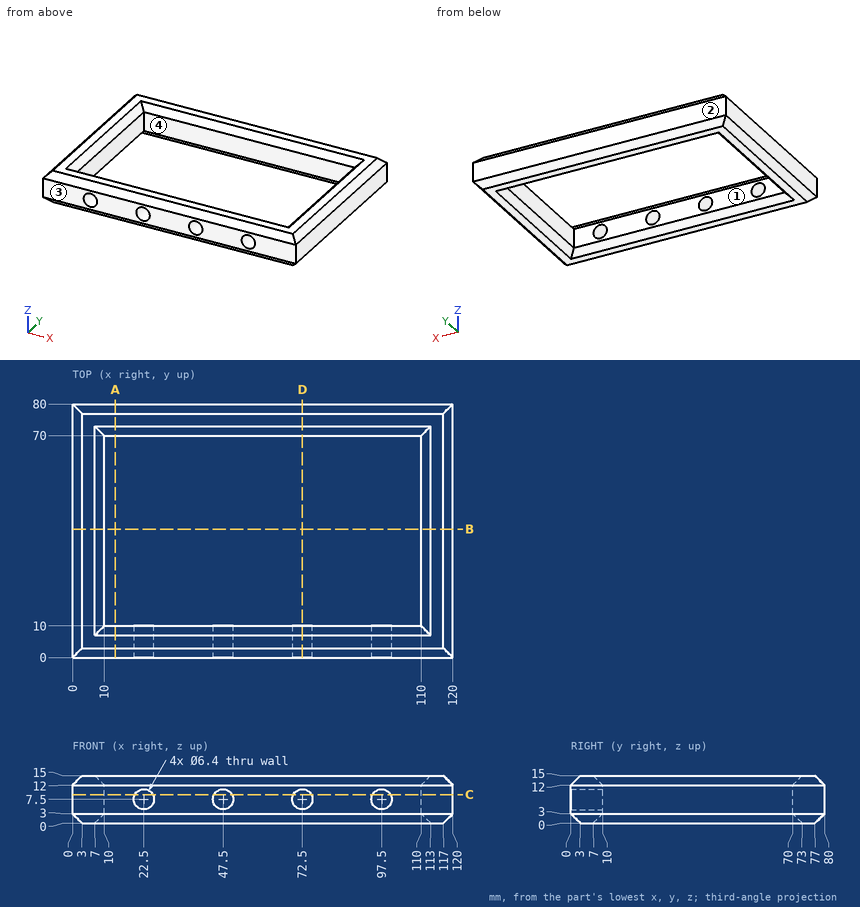
Answer from the drawing. Dimensions are ordinates in mm from the lowest x, y and z of the part. A direction names the side the tool comes from. Give positions to 0.01 mm unless a question says otherwise; leave off trailing zeros. Write each loop counter-clockwise with the first axis right and the second up, starting at its lowest first coordinate (ties: lowest second). Pieces come first, ordered by that corner, then holes.
1) Section B-B (y = 40.5) is taken. Write down the section's boundary in (x, z), and give its area (3 significant figures).
2) A tool of negligible diameter and unlimited length cuts with its end or side. For the marked faces 1 and 2, from which of +Z, -Z, +X, -X, +Y, -Y can it reach the whole face along a straight path? Write none if from no direction.
3) Find the intervals of material crossed by L1, parallel to X at y = 18, z = 5.75; L2, parallel to Y at x = 105, z = 6.75; L3, parallel to Z at x = 22.5, y = 6.25, in increasing order.
4) Given P1, Ø4, axis at x = 97.5, z = 7.5, coming from the -Y side, flat-ended and moving along its own axis, determine where the tip first touches the part or whether it passes through.
5) Section D-D (x = 72.5) is taken. Write down the section's boundary in (y, z), and give its area (3 significant figures).
6) For a pull along X with two mould halves and no side action, classify the marked faces 3 and 4 as pulls with the +X half, pulls with the -X half, needs draft (parallel to the pull), parting line crosses it, or undercut.
7) Section A-A (x = 13.5) is taken. Write down the section's boundary in (y, z), and give its area (3 significant figures).
8) Section C-C (z = 9) is taken. Write down the section's boundary in (x, y).
Response:
1. outline: (0, 3) - (3, 0) - (7, 0) - (10, 3) - (10, 12) - (7, 15) - (3, 15) - (0, 12) - close; (110, 3) - (113, 0) - (117, 0) - (120, 3) - (120, 12) - (117, 15) - (113, 15) - (110, 12) - close
1. area: 264 mm2
2. face 1: +Z, -Z
2. face 2: +Z, -Z, +X, -X, +Y
3. L1: x = 0 to 10, 110 to 120
3. L2: y = 0 to 10, 70 to 80
3. L3: z = 0 to 4.3, 10.7 to 15
4. P1: stops at y = 70
5. outline: (0, 3) - (3, 0) - (7, 0) - (10, 3) - (10, 4.3) - (0, 4.3) - close; (0, 10.7) - (10, 10.7) - (10, 12) - (7, 15) - (3, 15) - (0, 12) - close; (70, 3) - (73, 0) - (77, 0) - (80, 3) - (80, 12) - (77, 15) - (73, 15) - (70, 12) - close
5. area: 200 mm2
6. face 3: needs draft
6. face 4: undercut
7. outline: (0, 3) - (3, 0) - (7, 0) - (10, 3) - (10, 12) - (7, 15) - (3, 15) - (0, 12) - close; (70, 3) - (73, 0) - (77, 0) - (80, 3) - (80, 12) - (77, 15) - (73, 15) - (70, 12) - close
7. area: 264 mm2
8. outline: (0, 0) - (19.67, 0) - (19.67, 10) - (10, 10) - (10, 70) - (110, 70) - (110, 10) - (100.33, 10) - (100.33, 0) - (120, 0) - (120, 80) - (0, 80) - close; (25.33, 0) - (44.67, 0) - (44.67, 10) - (25.33, 10) - close; (50.33, 0) - (69.67, 0) - (69.67, 10) - (50.33, 10) - close; (75.33, 0) - (94.67, 0) - (94.67, 10) - (75.33, 10) - close
